```python
from build123d import *

# Parameters (mm, degrees)
SKETCH1_R           = 43.5
SKETCH1_R_2         = 35
BOSS_EXTRUDE1_DEPTH = 2
SKETCH2_R           = 1.5
CUT_EXTRUDE1_DEPTH  = 10
CIRPATTERN1_COUNT   = 12
CIRPATTERN2_COUNT   = 12


with BuildPart() as part:
    # Sketch1 → Boss-Extrude1 (new body)
    with BuildSketch(Plane.XY):
        Circle(SKETCH1_R)
        Circle(SKETCH1_R_2, mode=Mode.SUBTRACT)
    extrude(amount=BOSS_EXTRUDE1_DEPTH)

    # Sketch2 → Cut-Extrude1 (cut)
    with BuildSketch(Plane.XY.offset(2)):
        with Locations((0, 39)):
            Circle(SKETCH2_R)
    cut_extrude1 = extrude(amount=-CUT_EXTRUDE1_DEPTH, mode=Mode.SUBTRACT)

    # CirPattern1: Cut-Extrude1 ×12 about axis
    cirpattern1_axis = Axis((0, 0, 0), (0, 0, 1))
    for i in range(1, CIRPATTERN1_COUNT):
        add(cut_extrude1.rotate(cirpattern1_axis, i * 360 / CIRPATTERN1_COUNT), mode=Mode.SUBTRACT)

    # Sketch4 → CSK for M3 Flat Head Machine Screw1 (revolve, cut)
    with BuildSketch(Plane(origin=(0, 39, 2), x_dir=(0, -1, 0), z_dir=(1, 0, 0))):
        Polygon((0, 0), (0, 2), (1.6, 2), (1.6, 1.75), (3.35, 0), align=None)
    csk_for_m3_flat_head_machine_screw1 = revolve(axis=Axis((0, 39, 8.35), (0, 0, -1)), mode=Mode.SUBTRACT)

    # CirPattern2: CSK for M3 Flat Head Machine Screw1 ×12 about axis
    cirpattern2_axis = Axis((0, 0, 0), (0, 0, 1))
    for i in range(1, CIRPATTERN2_COUNT):
        add(csk_for_m3_flat_head_machine_screw1.rotate(cirpattern2_axis, i * 360 / CIRPATTERN2_COUNT), mode=Mode.SUBTRACT)


solid = part.part
```
For this review, take the finished solid that the model builds, in its own axes (mm). Round coordinates to 2 decimals unless told otherwise and drop trailing zeros. Order: outer loops, then holes, each group sorted by start corner. A loop starts at its lowest first (then second) coordinate and runs counter-clockwise, first axis right, second up.
Q1. We need section C-C, the plane z = 0.55. State how many separate pieces and enclosed holes the cut face has, plus the area to 3 significant figures.
Findings below:
separate pieces: 1
enclosed holes: 13
area: 1,960 mm2
Q2. We need section B-B, the plane x = -39. Give the boundary of the cut face in (y, z).
Findings below:
outline: (-19.27, 0) - (-1.6, 0) - (-1.6, 0.25) - (-3.35, 2) - (-19.27, 2) - close; (1.6, 0) - (19.27, 0) - (19.27, 2) - (3.35, 2) - (1.6, 0.25) - close
Q3. Mouldability with a two-part tool opening along X and no side actions: class faces 1 (the conical face through (19.28, -35.47, 0.36)), 2 (the flat face through (-20, 29, 2)) as pulls with the +X half, pulls with the -X half, needs draft (parallel to the pull), parting line crosses it, or undercut.
Findings below:
face 1: undercut
face 2: needs draft
Q4. Insertion check: P1, Ø5, axis at x = 19.5, y = 33.77, coming from the +Z side (3 decimals); P2, Ø2.5, axis at x = 33.77, y = -19.5, coming from the -Z side; P3, Ø8, axis at x = 34, y = 32.5, coming from the -Z side; P4, Ø1, axis at x = 21.5, z = 1, coming from the +Y side. Each pin has a flat end and moves straight along its axis. Give the tip position at first contact, or say it passes through.
Findings below:
P1: stops at z = 1.155
P2: passes through
P3: stops at z = 0
P4: stops at y = 38.1
Q5. Wall thickness on line 1 (Y direction, x = -19.5, z = 0.25) (3 decimals); line 2 (Y direction, x = -1, z = 0.1): over which ranges is each line inside the solid? List them lowest first.
Findings below:
line 1: y = -38.884 to -35.375, -32.175 to -29.065, 29.065 to 32.175, 35.375 to 38.884
line 2: y = -43.49 to -40.25, -37.75 to -34.99, 34.99 to 37.75, 40.25 to 43.49
Q6. We need section A-A, the plane x = 0. Give the boundary of the cut face in (y, z).
Findings below:
outline: (-43.5, 0) - (-40.6, 0) - (-40.6, 0.25) - (-42.35, 2) - (-43.5, 2) - close; (-37.4, 0) - (-35, 0) - (-35, 2) - (-35.65, 2) - (-37.4, 0.25) - close; (35, 0) - (37.4, 0) - (37.4, 0.25) - (35.65, 2) - (35, 2) - close; (40.6, 0) - (43.5, 0) - (43.5, 2) - (42.35, 2) - (40.6, 0.25) - close
